Check sheet for the drawn part. Datum: minimum x, y, z corner. Units: mm. A direction names the side the tool comes from. Round coordinates to 2 decimals unless told otherwise and drop trailing zeros. Write each loop counter-clockwise with the first axis right and the second up, starting at its lowest first coordinate (ties: lowest second). Pieces come first, ordered by that corner, then holes. Notation, with made-up numbers: (31.25, 79.5) - (85.25, 79.5) arc R24 cw to (85.25, 116.5) - close; hole circle Ø6 at (16.5, -16). An arc over 180 degrees is marked (long way). Return JSON: item names as keys, results as strings. Group by question number.
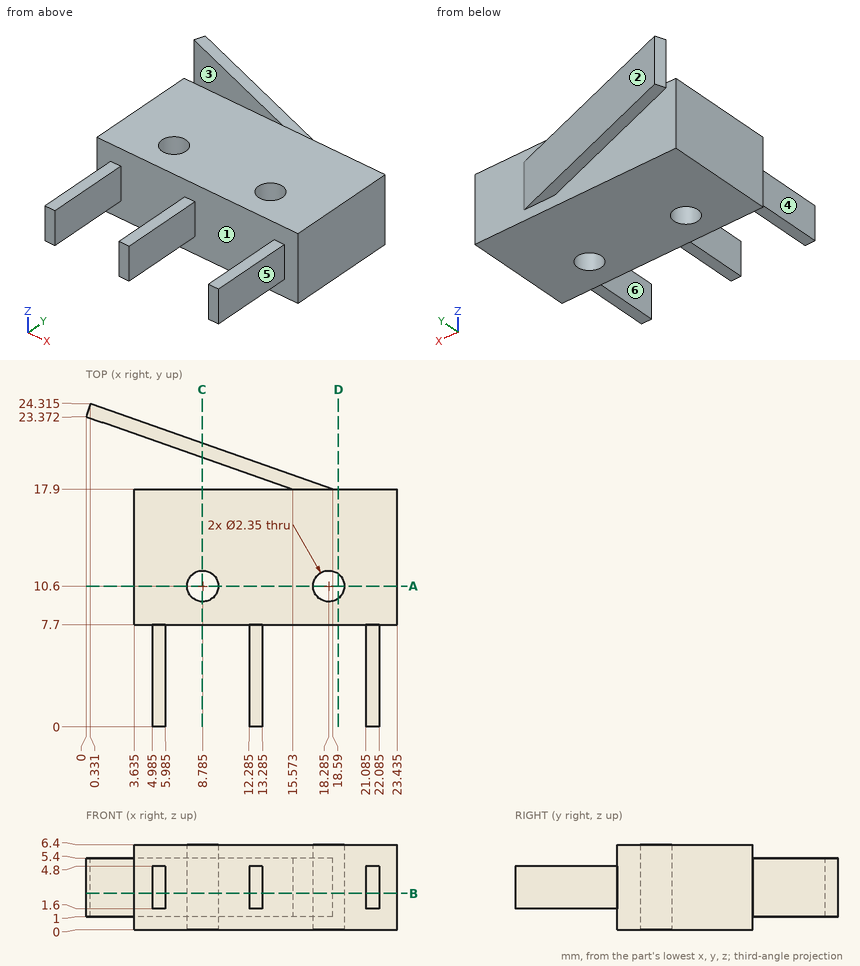
1. Mould release check, pull along X, two halves, no side actions. Record for the marked faces 1, 2 and 3: pulls with the +X half, pulls with the -X half, needs draft (parallel to the pull), parting line crosses it, or undercut.
2. Depth check by flat-ended pin: pin 1 Ø1 at (y, z) = (5.5, 3) entering from -X (1 decimal); pin 2 Ø0.5 at (x, y) = (21.5, 4) entering from -Z; pin 3 Ø2 at (x, y) = (5.5, 22) entering from +Z; pin 4 Ø1.9 at (x, y) = (18.28, 10.6) entering from -Z. Enter the tip coordinate at first touch or a pass-through.
3. Tool access check on the marked faces 4, 5 and 6. Record the directions out of +Z, -Z, +X, -X, +Y, -Y that give a thin tool (end or side, any length) a straight path to the whole face; none if there is none.
4. Section check B-B (z = 2.75). State how many separate pieces and enclosed holes the cut face has, and give its area (3 significant figures).
5. Section check A-A (y = 10.6). Enter the section's corners in (x, z) (1 decimal).
6. Section check D-D (x = 19). Enter the section's corners in (y, z).
7. Section check C-C (x = 8.75). Enter the section's corners in (y, z) (1 decimal).
8. Material ranges on line 1 along X through (y, z) = (10, 2.5) (1 decimal); line 2 along Y through (x, z) = (9.25, 4); line 3 along Y through (x, z) = (5.5, 5.75), recorded low to high.
Result sheet:
{
 "1": {"face 1": "undercut", "face 2": "pulls with the +X half", "face 3": "pulls with the -X half"},
 "2": {"pin 1": "stops at x = 5", "pin 2": "stops at z = 1.6", "pin 3": "stops at z = 5.4", "pin 4": "passes through"},
 "3": {"face 4": "+Z, -Z, -X, -Y", "face 5": "+Z, -Z, +X, -Y", "face 6": "+Z, -Z, -Y"},
 "4": {"separate pieces": "1", "enclosed holes": "2", "area": "234 mm²"},
 "5": {"outline": "(3.6, 0) - (7.6, 0) - (7.6, 6.4) - (3.6, 6.4) - close; (10, 0) - (17.1, 0) - (17.1, 6.4) - (10, 6.4) - close; (19.5, 0) - (23.4, 0) - (23.4, 6.4) - (19.5, 6.4) - close"},
 "6": {"outline": "(7.7, 0) - (9.67, 0) - (9.67, 6.4) - (7.7, 6.4) - close; (11.53, 0) - (17.9, 0) - (17.9, 6.4) - (11.53, 6.4) - close"},
 "7": {"outline": "(7.7, 0) - (9.4, 0) - (9.4, 6.4) - (7.7, 6.4) - close; (11.8, 0) - (17.9, 0) - (17.9, 6.4) - (11.8, 6.4) - close; (20.3, 1) - (21.4, 1) - (21.4, 5.4) - (20.3, 5.4) - close"},
 "8": {"line 1": "x = 3.6 to 7.8, 9.8 to 17.3, 19.3 to 23.4", "line 2": "y = 7.7 to 9.52, 11.68 to 17.9, 20.12 to 21.18", "line 3": "y = 7.7 to 17.9"}
}
